Input: part model. Units: mm. Frame: model coordinates. Round coordinates to 2 decimals unless told otherwise and drop trailing zeros. Order: outer loops, then holes, each group sorted by start corner. A loop starts at its lowest first (then second) coordinate and runs counter-clockwise, first axis right, second up.
Item 1: Cut plane B-B on x = -17. Output: boundary loops of the cut face in (y, z).
Item 2: Line query: L1, parallel to X at y = -1000, z = 5; L2, parallel to Y at x = -12, z = 6.25; L3, parallel to X at y = -873.5, z = 0.5. Output: solid intervals per line, ascending.
Item 3: Cut plane A-A on y = -1000. Output: boundary loops of the cut face in (x, z).
Item 4: First-contact query: pin 1 (6 mm diameter, centred on x = -36, y = -988, fed in from -Z); pin 2 (2.5 mm diameter, centred on y = -856, z = 5.5, fed in from +X); pin 3 (1 mm diameter, centred on y = -929.5, z = 4, fed in from -X). Flat tips, straight axial feed; report the tip coordinate or a pass-through.
Item 5: Cut plane C-C on y = -1088.5. Output: boundary loops of the cut face in (x, z).
Item 6: Cut plane D-D on z = 1.75. Give the number of separate pieces and of enclosed holes in the cut face, then the cut area to 3 significant figures.
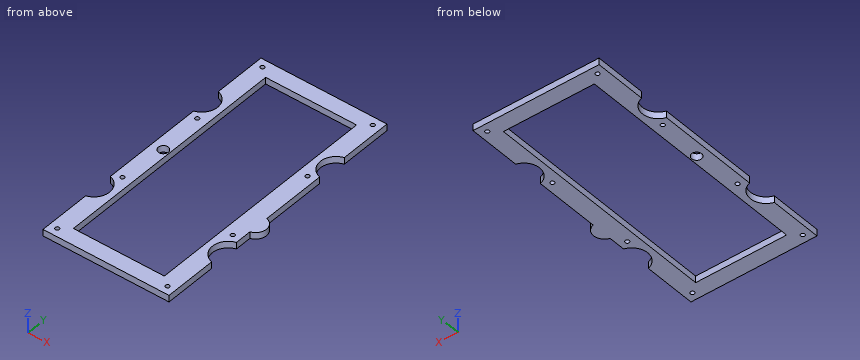
```python
from build123d import *

# Parameters (mm, degrees)
SKETCH1_R           = 2.5
BOSS_EXTRUDE1_DEPTH = 8
SKETCH5_W           = 110
SKETCH5_H           = 285
CUT_EXTRUDE4_DEPTH  = 9
SKETCH6_R           = 6
CUT_EXTRUDE5_DEPTH  = 9


with BuildPart() as part:
    # Sketch1 → Boss-Extrude1 (new body)
    with BuildSketch(Plane.XY):
        with BuildLine():
            Line((-61.080112923, -938.33030278), (-61.080112923, -1061.66969722))
            ThreePointArc((-61.080112923, -1061.66969722), (-47.080112923, -1080), (-61.080112923, -1098.33030278))
            Line((-61.080112923, -1098.33030278), (-61.080112923, -1161.56262))
            Line((-61.080112923, -1161.56262), (91.419887077, -1161.56262))
            Line((91.419887077, -1161.56262), (91.419887077, -1098.33030278))
            ThreePointArc((91.419887077, -1098.33030278), (77.419887077, -1080), (91.419887077, -1061.66969722))
            Line((91.419887077, -1061.66969722), (91.419887077, -1041.596868336))
            ThreePointArc((91.419887077, -1041.596868336), (101.085308187, -1029.0799835), (91.419887077, -1016.563098664))
            Line((91.419887077, -1016.563098664), (91.419887077, -938.33030278))
            ThreePointArc((91.419887077, -938.33030278), (77.419887077, -920), (91.419887077, -901.66969722))
            Line((91.419887077, -901.66969722), (91.419887077, -838.43738))
            Line((91.419887077, -838.43738), (-61.080112923, -838.43738))
            Line((-61.080112923, -838.43738), (-61.080112923, -901.66969722))
            ThreePointArc((-61.080112923, -901.66969722), (-47.080112923, -920), (-61.080112923, -938.33030278))
        make_face()
        with Locations((-51.580112923, -847.93738)):
            Circle(SKETCH1_R, mode=Mode.SUBTRACT)
        with Locations((81.919887077, -847.93738)):
            Circle(SKETCH1_R, mode=Mode.SUBTRACT)
        with Locations((81.919887077, -944.535688293)):
            Circle(SKETCH1_R, mode=Mode.SUBTRACT)
        with Locations((-51.580112923, -944.535688293)):
            Circle(SKETCH1_R, mode=Mode.SUBTRACT)
        with Locations((-51.580112923, -1055.464311707)):
            Circle(SKETCH1_R, mode=Mode.SUBTRACT)
        with Locations((81.919887077, -1055.464311707)):
            Circle(SKETCH1_R, mode=Mode.SUBTRACT)
        with Locations((81.919887077, -1152.06262)):
            Circle(SKETCH1_R, mode=Mode.SUBTRACT)
        with Locations((-51.580112923, -1152.06262)):
            Circle(SKETCH1_R, mode=Mode.SUBTRACT)
    extrude(amount=BOSS_EXTRUDE1_DEPTH)

    # Sketch5 → Cut-Extrude4 (cut, through all)
    with BuildSketch(Plane(origin=(0, 0, 0), x_dir=(-1, 0, 0), z_dir=(0, 0, -1))):
        with Locations((-15.169887077, -1000)):
            Rectangle(SKETCH5_W, SKETCH5_H)
    extrude(amount=-CUT_EXTRUDE4_DEPTH, mode=Mode.SUBTRACT)

    # Sketch6 → Cut-Extrude5 (cut, through all)
    with BuildSketch(Plane.XY.offset(8)):
        with Locations((-47.330112923, -1000)):
            Circle(SKETCH6_R)
    extrude(amount=-CUT_EXTRUDE5_DEPTH, mode=Mode.SUBTRACT)


solid = part.part
```
From the geometry:
1. outline: (-1161.56, 0) - (-1142.5, 0) - (-1142.5, 8) - (-1161.56, 8) - close; (-857.5, 0) - (-838.44, 0) - (-838.44, 8) - (-857.5, 8) - close
2. L1: x = -61.08 to -53.33, -41.33 to -39.83, 70.17 to 91.42
2. L2: y = -1161.56 to -1142.5, -857.5 to -838.44
2. L3: x = -61.08 to -39.83, 70.17 to 91.42
3. outline: (-61.08, 0) - (-53.33, 0) - (-53.33, 8) - (-61.08, 8) - close; (-41.33, 0) - (-39.83, 0) - (-39.83, 8) - (-41.33, 8) - close; (70.17, 0) - (91.42, 0) - (91.42, 8) - (70.17, 8) - close
4. pin 1: passes through
4. pin 2: stops at x = 91.42
4. pin 3: stops at x = -49.92
5. outline: (-49.09, 0) - (-39.83, 0) - (-39.83, 8) - (-49.09, 8) - close; (70.17, 0) - (79.43, 0) - (79.43, 8) - (70.17, 8) - close
6. separate pieces: 1
6. enclosed holes: 10
6. area: 16,300 mm2
